Read the model definition and answer for the solid it produces. Units are mm, in the model's axes. Give positions to 0.01 mm unless a question says otherwise; leave off trailing zeros. Loops run counter-clockwise (first coordinate to the right, second up) from the corner with the lowest first, then second, coordinate; pieces in that order, holes last. Notation, with made-up numbers: (34.5, 40.5) - (38.5, 40.5) arc R27 cw to (38.5, 76.5) - close; hole circle Ø3 at (3.25, 9.25). An arc over 180 degrees is marked (long way). Write item = value, one per line.
```python
from build123d import *

# Parameters (mm, degrees)
SKETCH1_R           = 3.55
SKETCH1_R_2         = 2.6
BOSS_EXTRUDE1_DEPTH = 3


with BuildPart() as part:
    # Sketch1 → Boss-Extrude1 (new body)
    with BuildSketch(Plane(origin=(0, 0, 0), x_dir=(1, 0, 0), z_dir=(0, 1, 0))):
        with BuildLine():
            Line((50, -70), (-50, -70))
            ThreePointArc((-50, -70), (-57.071067812, -67.071067812), (-60, -60))
            Line((-60, -60), (-60, 60))
            ThreePointArc((-60, 60), (-57.071067812, 67.071067812), (-50, 70))
            Line((-50, 70), (50, 70))
            ThreePointArc((50, 70), (57.071067812, 67.071067812), (60, 60))
            Line((60, 60), (60, -60))
            ThreePointArc((60, -60), (57.071067812, -67.071067812), (50, -70))
        make_face()
        with Locations((-32.3, 52.3)):
            Circle(SKETCH1_R, mode=Mode.SUBTRACT)
        with Locations((0, 10)):
            Circle(SKETCH1_R_2, mode=Mode.SUBTRACT)
        Circle(SKETCH1_R_2, mode=Mode.SUBTRACT)
        with Locations((10, 0)):
            Circle(SKETCH1_R_2, mode=Mode.SUBTRACT)
        with Locations((-10, 0)):
            Circle(SKETCH1_R_2, mode=Mode.SUBTRACT)
        with Locations((-42.3, 52.3)):
            Circle(SKETCH1_R, mode=Mode.SUBTRACT)
        with Locations((-42.3, 0)):
            Circle(SKETCH1_R, mode=Mode.SUBTRACT)
        with Locations((-42.3, -52.3)):
            Circle(SKETCH1_R, mode=Mode.SUBTRACT)
        with Locations((-30, 20)):
            Circle(SKETCH1_R_2, mode=Mode.SUBTRACT)
        with Locations((-45, 10)):
            Circle(SKETCH1_R_2, mode=Mode.SUBTRACT)
        with Locations((-20, 30)):
            Circle(SKETCH1_R_2, mode=Mode.SUBTRACT)
        with Locations((0, 20)):
            Circle(SKETCH1_R_2, mode=Mode.SUBTRACT)
        with Locations((-10, 52.3)):
            Circle(SKETCH1_R_2, mode=Mode.SUBTRACT)
        with Locations((0, 52.3)):
            Circle(SKETCH1_R_2, mode=Mode.SUBTRACT)
        with Locations((10, 52.3)):
            Circle(SKETCH1_R_2, mode=Mode.SUBTRACT)
        with Locations((0, 30)):
            Circle(SKETCH1_R_2, mode=Mode.SUBTRACT)
        with Locations((20, 30)):
            Circle(SKETCH1_R_2, mode=Mode.SUBTRACT)
        with Locations((30, 20)):
            Circle(SKETCH1_R_2, mode=Mode.SUBTRACT)
        with Locations((45, 10)):
            Circle(SKETCH1_R_2, mode=Mode.SUBTRACT)
        with Locations((32.3, 52.3)):
            Circle(SKETCH1_R_2, mode=Mode.SUBTRACT)
        with Locations((42.3, 52.3)):
            Circle(SKETCH1_R_2, mode=Mode.SUBTRACT)
        with Locations((42.3, 0)):
            Circle(SKETCH1_R_2, mode=Mode.SUBTRACT)
        with Locations((45, -10)):
            Circle(SKETCH1_R_2, mode=Mode.SUBTRACT)
        with Locations((42.3, -52.3)):
            Circle(SKETCH1_R_2, mode=Mode.SUBTRACT)
        with Locations((32.3, -52.3)):
            Circle(SKETCH1_R_2, mode=Mode.SUBTRACT)
        with Locations((30, -20)):
            Circle(SKETCH1_R_2, mode=Mode.SUBTRACT)
        with Locations((0, -10)):
            Circle(SKETCH1_R_2, mode=Mode.SUBTRACT)
        with Locations((20, -30)):
            Circle(SKETCH1_R_2, mode=Mode.SUBTRACT)
        with Locations((20, 0)):
            Circle(SKETCH1_R_2, mode=Mode.SUBTRACT)
        with Locations((10, -52.3)):
            Circle(SKETCH1_R_2, mode=Mode.SUBTRACT)
        with Locations((0, -52.3)):
            Circle(SKETCH1_R_2, mode=Mode.SUBTRACT)
        with Locations((-10, -52.3)):
            Circle(SKETCH1_R_2, mode=Mode.SUBTRACT)
        with Locations((30, 0)):
            Circle(SKETCH1_R_2, mode=Mode.SUBTRACT)
        with Locations((-20, -30)):
            Circle(SKETCH1_R_2, mode=Mode.SUBTRACT)
        with Locations((-30, -20)):
            Circle(SKETCH1_R_2, mode=Mode.SUBTRACT)
        with Locations((-45, -10)):
            Circle(SKETCH1_R_2, mode=Mode.SUBTRACT)
        with Locations((-32.3, -52.3)):
            Circle(SKETCH1_R, mode=Mode.SUBTRACT)
        with Locations((-22.3, 52.3)):
            Circle(SKETCH1_R, mode=Mode.SUBTRACT)
        with Locations((22.3, 52.3)):
            Circle(SKETCH1_R_2, mode=Mode.SUBTRACT)
        with Locations((-20, 0)):
            Circle(SKETCH1_R_2, mode=Mode.SUBTRACT)
        with Locations((-30, 0)):
            Circle(SKETCH1_R_2, mode=Mode.SUBTRACT)
        with Locations((-42.3, 26.3)):
            Circle(SKETCH1_R, mode=Mode.SUBTRACT)
        with Locations((22.3, -52.3)):
            Circle(SKETCH1_R_2, mode=Mode.SUBTRACT)
        with Locations((-22.3, -52.3)):
            Circle(SKETCH1_R, mode=Mode.SUBTRACT)
        with Locations((-42.3, -26.3)):
            Circle(SKETCH1_R, mode=Mode.SUBTRACT)
        with Locations((42.3, 26.3)):
            Circle(SKETCH1_R_2, mode=Mode.SUBTRACT)
        with Locations((42.3, -26.3)):
            Circle(SKETCH1_R_2, mode=Mode.SUBTRACT)
        with Locations((0, -30)):
            Circle(SKETCH1_R_2, mode=Mode.SUBTRACT)
        with Locations((0, -20)):
            Circle(SKETCH1_R_2, mode=Mode.SUBTRACT)
    extrude(amount=BOSS_EXTRUDE1_DEPTH)


solid = part.part
```
1) A cutting plane is placed at C-C on z = 52.3. Give the number of separate pieces and of enclosed holes in the cut face, then the cut area to 4 significant figures.
Output:
separate_pieces = 10
enclosed_holes = 0
area = 202.5 mm²
2) The mould has two halves that part along Z. Classify faces 1 (the face through (-38.914, 1.479, -27.366)), 2 (the face through (-1, 1, -70)), 3 (the face through (57.15, 1.48, 66.99)): pulls with the +Z half, pulls with the -Z half, needs draft (parallel to the pull), parting line crosses it, or undercut.
Output:
face_1 = undercut
face_2 = pulls with the -Z half
face_3 = pulls with the +Z half
3) A cutting plane is placed at A-A on x = -10. Determine the outline of the cut face in (y, z).
Output:
outline = (0, -70) - (3, -70) - (3, -54.9) - (0, -54.9) - close; (0, -49.7) - (3, -49.7) - (3, -2.6) - (0, -2.6) - close; (0, 2.6) - (3, 2.6) - (3, 49.7) - (0, 49.7) - close; (0, 54.9) - (3, 54.9) - (3, 70) - (0, 70) - close
4) Find the intervals of material crossed by probe 1 along Z at (x, y) = (-42.3, 1.6); probe 2 along X at (y, z) = (0.7, 10); probe 3 along Z at (x, y) = (34, 2.7), in increasing order.
Output:
probe_1 = -70 to -55.85, -48.75 to -29.85, -22.75 to -3.55, 3.55 to 22.75, 29.85 to 48.75, 55.85 to 70
probe_2 = -60 to -47.6, -42.4 to -2.6, 2.6 to 42.4, 47.6 to 60
probe_3 = -70 to -54.27, -50.33 to 50.33, 54.27 to 70
5) This flat-tipped pin is pushed along its axis until it touches: P1, Ø4.5, axis at x = 0, z = 20, coming from the -Y side. Where does it stop, or does it pass through?
Output:
P1 = through
6) A cutting plane is placed at B-B on z = -20. Determine the outline of the cut face in (x, y), then the cut area to 3 significant figures.
Output:
outline = (-60, 0) - (-32.6, 0) - (-32.6, 3) - (-60, 3) - close; (-27.4, 0) - (-2.6, 0) - (-2.6, 3) - (-27.4, 3) - close; (2.6, 0) - (27.4, 0) - (27.4, 3) - (2.6, 3) - close; (32.6, 0) - (60, 0) - (60, 3) - (32.6, 3) - close
area = 313 mm²
